Input: part model. Units: mm. Frame: model coordinates. A direction names the side the tool comes from. Coordinates: 2 decimals unless noted, no trailing zeros. Write each loop counter-clockwise with the first axis right and the second up, starting at its lowest first coordinate (ties: lowest second). Pieces come first, ordered by that corner, then holes.
1) Section query B-B (z = 0). Output: boundary loops of the cut face in (x, y), then the cut area to 3 significant figures.
2) Section query C-C (x = 0). Output: boundary loops of the cut face in (y, z), then the cut area to 3 significant figures.
3) Line query: L1, parallel to Z at x = -6, y = 5; L2, parallel to Y at x = 2.5, z = 5.25; L3, parallel to X at y = 2.3, z = 0. Output: solid intervals per line, ascending.
4) Section query A-A (y = 17). Output: boundary loops of the cut face in (x, z), then the cut area to 3 significant figures.
5) Section query D-D (y = 47). Output: boundary loops of the cut face in (x, z).
6) Pin query (flat end, axial travel): pin 1 Ø7 at (x, z) = (0, 0) entering from +Y; pin 2 Ø2 at (y, z) = (9.5, 0) entering from -X; pin 3 Ø12 at (y, z) = (18, 7) entering from +X; pin 4 Ø4 at (y, z) = (16.5, -1.5) entering from +X. Return the tip coordinate at first contact, or that it passes through.
7) Draft query along Y for faces 1 (the flat face through (-4, 0, 0)), 2 (the flat face through (-5, 17, 10)), 3 (the flat face through (-13, 25, 2.7)). Return one class per face: pulls with the +Y half, pulls with the -Y half, needs draft (parallel to the pull), parting line crosses it, or undercut.
8) Set-up query: faces 4 (the cylindrical face through (-2.685, 1.479, -0.596)), 5 (the flat face through (-13, 26, -2.7)), 6 (the flat face through (4, 3, 0)). Return all of +Z, -Z, +X, -X, +Y, -Y with unobstructed straight access to the full face (end or side cutting, diameter ignored); none if empty.
from build123d import *

# Parameters (mm, degrees)
SKETCH1_W           = 30
SKETCH1_H           = 20
SKETCH1_R           = 2.75
BOSS_EXTRUDE1_DEPTH = 3
SKETCH2_W           = 3
SKETCH2_H           = 20
BOSS_EXTRUDE2_DEPTH = 50
RIB1_REACH          = 60.6
SKETCH3_WALL_W      = 176.024973172
SKETCH3_WALL_H      = 3
CUT_EXTRUDE1_DEPTH  = 61.3158354


with BuildPart() as part:
    # Sketch1 → Boss-Extrude1 (new body)
    with BuildSketch(Plane(origin=(0, 0, 0), x_dir=(1, 0, 0), z_dir=(0, 1, 0))):
        Rectangle(SKETCH1_W, SKETCH1_H)
        with Locations(Location((0, 0, 0), (0, 0, 270))):
            Circle(SKETCH1_R, mode=Mode.SUBTRACT)
    extrude(amount=BOSS_EXTRUDE1_DEPTH)

    # Sketch2 → Boss-Extrude2 (add)
    with BuildSketch(Plane(origin=(0, 3, 0), x_dir=(1, 0, 0), z_dir=(0, 1, 0))):
        with Locations((-13.5, 0)):
            Rectangle(SKETCH2_W, SKETCH2_H)
    extrude(amount=BOSS_EXTRUDE2_DEPTH)

    # Sketch3 wall → Rib1 (add, up to next)
    with BuildSketch(Plane(origin=(1.5, 28, 10), x_dir=(0.475148914735, -0.879905397657, 0), z_dir=(0.879905397657, 0.475148914735, 0)), mode=Mode.PRIVATE) as rib1_sk1:
        with Locations((0, 1.5)):
            Rectangle(SKETCH3_WALL_W, SKETCH3_WALL_H)
    rib1_tool1 = extrude(rib1_sk1.sketch, amount=-RIB1_REACH, mode=Mode.PRIVATE) - part.part
    rib1 = rib1_tool1.solids().sort_by_distance((1.5, 28, 10))[0]
    add(rib1)

    # Mirror1: Rib1 across plane
    add(rib1.mirror(Plane.XY))

    # Sketch4 → Cut-Extrude1 (cut, through all)
    with BuildSketch(Plane(origin=(-12, 0, 0), x_dir=(0, 0, -1), z_dir=(1, 0, 0))):
        with BuildLine():
            Line((2.7, 43), (2.7, 8))
            ThreePointArc((2.7, 8), (0, 5.3), (-2.7, 8))
            Line((-2.7, 8), (-2.7, 43))
            ThreePointArc((-2.7, 43), (0, 45.7), (2.7, 43))
        make_face()
    extrude(amount=-CUT_EXTRUDE1_DEPTH, mode=Mode.SUBTRACT)


solid = part.part
Answer:
1. outline: (-15, 0) - (-2.75, 0) - (-2.75, 3) - (-12, 3) - (-12, 5.3) - (-15, 5.3) - close; (-15, 45.7) - (-12, 45.7) - (-12, 53) - (-15, 53) - close; (2.75, 0) - (15, 0) - (15, 3) - (2.75, 3) - close
1. area: 102 mm2
2. outline: (0, -10) - (30.78, -10) - (30.78, -7) - (3, -7) - (3, -2.75) - (0, -2.75) - close; (0, 2.75) - (3, 2.75) - (3, 7) - (30.78, 7) - (30.78, 10) - (0, 10) - close
2. area: 210 mm2
3. L1: z = -10 to -7, 7 to 10
3. L2: y = 0 to 3
3. L3: x = -15 to -2.75, 2.75 to 15
4. outline: (-15, -10) - (7.44, -10) - (7.44, -7) - (-12, -7) - (-12, -2.7) - (-15, -2.7) - close; (-15, 2.7) - (-12, 2.7) - (-12, 7) - (7.44, 7) - (7.44, 10) - (-15, 10) - close
4. area: 160 mm2
5. outline: (-15, -10) - (-8.76, -10) - (-8.76, -7) - (-12, -7) - (-12, 7) - (-8.76, 7) - (-8.76, 10) - (-15, 10) - close
6. pin 1: stops at y = 3
6. pin 2: passes through
6. pin 3: stops at x = 10.14
6. pin 4: stops at x = -12
7. face 1: pulls with the -Y half
7. face 2: needs draft
7. face 3: undercut
8. face 4: +Y, -Y
8. face 5: +X, -X
8. face 6: +X, +Y
